Model file for the job. Use its own axes, mm. A direction names the side the tool comes from. Give positions to 0.01 mm unless a question says otherwise; leave off trailing zeros. Loops run counter-clockwise (first coordinate to the right, second up) from the corner with the lowest first, then second, coordinate; pieces in that order, holes last. Notation, with made-up numbers: M 53.5,-35.75 L 93.5,-35.75 A21 ccw 93.5,-2.75 Z; hole C 56.5,-22.5 d7. An arc over 180 degrees is marked long. Answer in a Markdown table with one row per item.
```python
from build123d import *

# Parameters (mm, degrees)
SKETCH2_W           = 29.5
SKETCH2_H           = 39
BOSS_EXTRUDE1_DEPTH = 6
SKETCH3_R           = 10.25
CUT_EXTRUDE1_DEPTH  = 3.5
SKETCH4_R           = 1.75
CUT_EXTRUDE2_DEPTH  = 3.5
SKETCH5_R           = 3.6
CUT_EXTRUDE3_DEPTH  = 9.9
SKETCH6_R           = 3.6
CUT_EXTRUDE4_DEPTH  = 9.9
SKETCH7_R           = 3.5
BOSS_EXTRUDE2_DEPTH = 9.7
CUT_EXTRUDE5_REACH  = 21.6
SKETCH8_R           = 1.45
SKETCH9_W           = 10
SKETCH9_H           = 2
BOSS_EXTRUDE3_DEPTH = 0.8
FILLET1_R           = 0.5


with BuildPart() as part:
    # Sketch2 → Boss-Extrude1 (new body)
    with BuildSketch(Plane(origin=(0, 0, 0), x_dir=(1, 0, 0), z_dir=(0, 1, 0))):
        with Locations((3.309391497, -2.30838063)):
            Rectangle(SKETCH2_W, SKETCH2_H)
    extrude(amount=BOSS_EXTRUDE1_DEPTH)

    # Sketch3 → Cut-Extrude1 (cut)
    with BuildSketch(Plane(origin=(0, 6, 0), x_dir=(1, 0, 0), z_dir=(0, 1, 0))):
        with Locations((3.309391497, -7.038449274)):
            Circle(SKETCH3_R)
    extrude(amount=-CUT_EXTRUDE1_DEPTH, mode=Mode.SUBTRACT)

    # Sketch4 → Cut-Extrude2 (cut, through all)
    with BuildSketch(Plane(origin=(0, 2.5, 0), x_dir=(1, 0, 0), z_dir=(0, 1, 0))):
        with Locations((3.309391497, -7.038449274)):
            Circle(SKETCH4_R)
    extrude(amount=-CUT_EXTRUDE2_DEPTH, mode=Mode.SUBTRACT)

    # Sketch5 → Cut-Extrude3 (cut)
    with BuildSketch(Plane(origin=(18.059391497, 0, 0), x_dir=(0, 0, -1), z_dir=(1, 0, 0))):
        with Locations((17.19161937, 6)):
            Circle(SKETCH5_R)
    extrude(amount=-CUT_EXTRUDE3_DEPTH, mode=Mode.SUBTRACT)

    # Sketch6 → Cut-Extrude4 (cut)
    with BuildSketch(Plane.ZY.offset(11.440608503)):
        with Locations((-17.19161937, 6)):
            Circle(SKETCH6_R)
    extrude(amount=-CUT_EXTRUDE4_DEPTH, mode=Mode.SUBTRACT)

    # Sketch7 → Boss-Extrude2 (add)
    with BuildSketch(Plane.ZY.offset(1.540608503)):
        with Locations((-17.19161937, 6)):
            Circle(SKETCH7_R)
    extrude(amount=-BOSS_EXTRUDE2_DEPTH)

    # Sketch8 → Cut-Extrude5 (cut, up to next)
    with BuildSketch(Plane(origin=(8.159391497, 0, 0), x_dir=(0, 0, -1), z_dir=(1, 0, 0)), mode=Mode.PRIVATE) as cut_extrude5_sk1:
        with Locations((17.19161937, 6)):
            Circle(SKETCH8_R)
    cut_extrude5_tool1 = extrude(cut_extrude5_sk1.sketch, amount=-CUT_EXTRUDE5_REACH, mode=Mode.PRIVATE) & part.part
    add(cut_extrude5_tool1.solids().sort_by_distance((8.159391, 6, -17.191619))[0], mode=Mode.SUBTRACT)

    # Sketch9 → Boss-Extrude3 (add)
    with BuildSketch(Plane.XY.offset(21.80838063)):
        with Locations((3.309391497, 5)):
            Rectangle(SKETCH9_W, SKETCH9_H)
    extrude(amount=BOSS_EXTRUDE3_DEPTH)

    # Fillet1
    fillet1_edges = [part.edges().sort_by_distance(p)[0] for p in [
        (-1.690608503, 5, 22.60838063),
        (3.309391497, 4, 22.60838063),
        (8.309391497, 5, 22.60838063),
        (3.309391497, 6, 22.60838063),
    ]]
    fillet(fillet1_edges, radius=FILLET1_R)


solid = part.part
```
(1) Saw through at B-B, the plane x = 16.25. Give the cut face in (y, z).
Established:
| item | result |
|---|---|
| outline | M 0,-17.19 L 2.4,-17.19 A3.6 cw 6,-13.59 L 6,21.81 L 0,21.81 Z |
(2) Mould opens along Z. For faces 5 (the cylindrical face through (3.24, 8.56, -19.58)), 6 (the cylindrical face through (3.377, 6.98, -16.123)), 7 (the flat face through (8.159, 4, -17)), 8 (the cylindrical face through (13.2, 3.5, -14.6)) say: pulls with the +Z half, pulls with the -Z half, needs draft (parallel to the pull), parting line crosses it, or undercut.
Established:
| item | result |
|---|---|
| face 5 | parting line crosses it |
| face 6 | undercut |
| face 7 | needs draft |
| face 8 | pulls with the -Z half |
(3) Which spindle directions (+Z, -Z, +X, -X, +Y, -Y) get a long thin tool onto all of the face, cutting with end or side? Do faces 1 (the cylindrical face through (-6.6, 3.4, -14.7)), 2 (the flat face through (3, 6, -4)), 3 (the flat face through (3, 1, -17.192)), 4 (the flat face through (5.4, 2.5, 6.9)). Say none if no direction does.
Established:
| item | result |
|---|---|
| face 1 | -Z, -X, +Y |
| face 2 | +Z, +X, -X, +Y |
| face 3 | -Z, +X, -X, -Y |
| face 4 | +Y |
(4) Saw through at D-D, the plane x = -4.5. Give the cut face in (y, z), and give its area (3 significant figures).
Established:
| item | result |
|---|---|
| outline | M 0,-17.19 L 2.4,-17.19 A3.6 cw 6,-13.59 L 6,0.4 L 2.5,0.4 L 2.5,13.68 L 6,13.68 L 6,21.81 L 0,21.81 Z |
| area | 177 mm2 |
(5) Saw through at A-A, the plane y = 6.75. Give the cut face in (x, z), and give its area (3 significant figures).
Established:
| item | result |
|---|---|
| outline | M -1.54,-20.61 L 8.16,-20.61 L 8.16,-18.43 L -1.54,-18.43 Z; M -1.54,-15.95 L 8.16,-15.95 L 8.16,-13.77 L -1.54,-13.77 Z |
| area | 42.2 mm2 |
(6) Flat gauge pins, fed straight in: P1, Ø2, axis at x = 3.31, z = 7.04, coming from the +Y side; P2, Ø4, axis at x = 13.5, y = 3.5, coming from the +Z side; P3, Ø3, axis at x = 9, y = 2, coming from the -Z side. Where does each tip first touch, or does it go through?
Established:
| item | result |
|---|---|
| P1 | passes through |
| P2 | stops at z = 21.81 |
| P3 | stops at z = -19.35 |
(7) Saw through at C-C, the plane z = 15. Give the cut face in (x, y).
Established:
| item | result |
|---|---|
| outline | M -11.44,0 L 18.06,0 L 18.06,6 L 9.77,6 L 9.77,2.5 L -3.15,2.5 L -3.15,6 L -11.44,6 Z |
(8) Wall check: L1, parallel to Z at x = 7, y = 5; L2, parallel to Y at x = 11.25, z = 5.5; L3, parallel to X at y = 4, z = -18.5. Give the ranges that are in metal, low to high.
Established:
| item | result |
|---|---|
| L1 | z = -20.55 to -18.24, -16.14 to -2.52, 16.6 to 22.61 |
| L2 | y = 0 to 2.5 |
| L3 | x = -1.54 to 8.16 |
